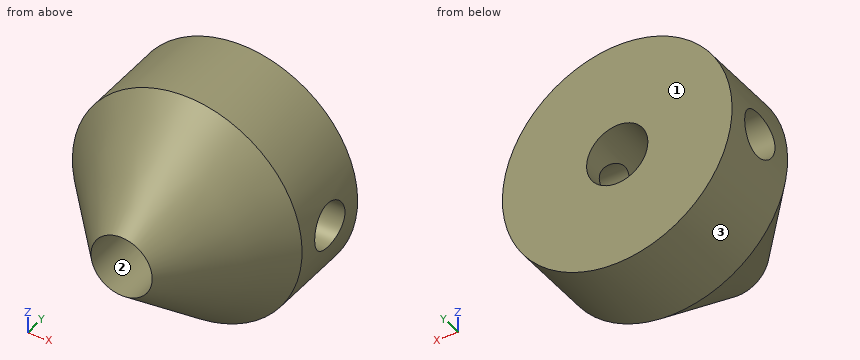
from build123d import *

# Parameters (mm, degrees)
CUT_EXTRUDE1_DEPTH      = 17.015617378
CUT_EXTRUDE1_DEPTH_BACK = 17.015617378
SKETCH2_R               = 1.5
SKETCH3_R               = 2
CUT_EXTRUDE2_DEPTH      = 17.015617484


with BuildPart() as part:
    # Sketch1 → Revolve1 (revolve)
    with BuildSketch(Plane(origin=(0, 0, 0), x_dir=(0, 0, -1), z_dir=(1, 0, 0)), mode=Mode.PRIVATE) as revolve1_sk:
        Polygon((0, 0), (-7.5, 0), (-7.5, -5.5), (-2, -12), (0, -12), align=None)
    revolve(revolve1_sk.sketch.rotate(Axis((0, -12, 0), (0, 1, 0)), 180), axis=Axis((0, -12, 0), (0, 1, 0)))

    # Sketch2 → Cut-Extrude1 (cut, two sides: drawn at the far end of the back side and taken through both)
    with BuildSketch(Plane(origin=(0, 0, 0), x_dir=(0, 0, -1), z_dir=(1, 0, 0)).offset(-CUT_EXTRUDE1_DEPTH_BACK)):
        with Locations((0, -2.75)):
            Circle(SKETCH2_R)
    extrude(amount=CUT_EXTRUDE1_DEPTH + CUT_EXTRUDE1_DEPTH_BACK, mode=Mode.SUBTRACT)

    # Sketch3 → Cut-Extrude2 (cut, through all)
    with BuildSketch(Plane(origin=(0, 0, 0), x_dir=(1, 0, 0), z_dir=(0, 1, 0))):
        with Locations(Location((0, 0, 0), (0, 0, 270))):
            Circle(SKETCH3_R)
    extrude(amount=-CUT_EXTRUDE2_DEPTH, mode=Mode.SUBTRACT)


solid = part.part
Input: part model. Units: mm. Frame: model coordinates. Face numbers are marked on the shaded views. Give positions to 0.01 mm unless a question says otherwise; leave off trailing zeros. Order: outer loops, then holes, each group sorted by start corner. A loop starts at its lowest first (then second) coordinate and runs counter-clockwise, first axis right, second up.
Q1. Section A-A on z = 0. Output: boundary loops of the cut face in (x, y), and give its area (4 significant figures).
Checked values:
outline: (-7.5, -5.5) - (-2, -12) - (-2, -4.25) - (-7.5, -4.25) - close; (-7.5, -1.25) - (-2, -1.25) - (-2, 0) - (-7.5, 0) - close; (2, -12) - (7.5, -5.5) - (7.5, -4.25) - (2, -4.25) - close; (2, -1.25) - (7.5, -1.25) - (7.5, 0) - (2, 0) - close
area: 63.25 mm2
Q2. Section B-B on x = 0. Output: boundary loops of the cut face in (y, z).
Checked values:
outline: (-12, -2) - (-5.5, -7.5) - (0, -7.5) - (0, -2) - close; (-12, 2) - (0, 2) - (0, 7.5) - (-5.5, 7.5) - close
Q3. Draft query along Z for the marked faces 1, 2 and 3. Return one class per face: +Z half, -Z half, draft (parallel to the pull), parting line (faces both ways), or undercut.
Checked values:
face 1: draft
face 2: undercut
face 3: parting line
Q4. Section D-D on y = -6.25. Output: boundary loops of the cut face in (x, z), and give its area (3 significant figures).
Checked values:
outline: circle Ø13.73 at (0, 0); hole circle Ø4 at (0, 0)
area: 136 mm2
Q5. Contact query for flat-ended pins moving along their axis: pin 1 Ø5 at (y, z) = (-3, 5) entering from +X; pin 2 Ø4 at (x, z) = (5.5, -5) entering from -Y; pin 3 Ø1 at (x, y) = (3.5, -7.5) entering from +Z. Output: stop coordinate, or through.
Checked values:
pin 1: stops at x = 7.07
pin 2: stops at y = -7.94
pin 3: stops at z = 5.25
Q6. Ray query, probe 1 along X at (y, z) = (-5.25, 0); probe 2 along Y at (x, z) = (4.25, 0); probe 3 along X at (y, z) = (-6, -1.5). Return the intervals inside material, ascending.
Checked values:
probe 1: x = -7.5 to -2, 2 to 7.5
probe 2: y = -9.34 to -4.25, -1.25 to 0
probe 3: x = -6.92 to -1.32, 1.32 to 6.92
Q7. Section C-C on y = -1.75. Output: boundary loops of the cut face in (x, z).
Checked values:
outline: (-7.42, -1.12) arc R7.5 ccw to (7.42, -1.12) - (1.66, -1.12) arc R2 cw to (-1.66, -1.12) - close; (-7.42, 1.12) - (-1.66, 1.12) arc R2 cw to (1.66, 1.12) - (7.42, 1.12) arc R7.5 ccw to start
